```python
from build123d import *

# Parameters (mm, degrees)
SKETCH_1_R          = 1.65
EXTRUDE_1_DEPTH     = 4
CUT_EXTRUDE_1_DEPTH = 2
SKETCH_5_R          = 3.15
SKETCH_5_R_2        = 1.65
EXTRUDE_3_DEPTH     = 2.5
EXTRUDE_2_DEPTH     = 14.5
SKETCH_4_R          = 1.15
CUT_EXTRUDE_2_DEPTH = 13.5
CUT_EXTRUDE_3_DEPTH = 8.5
EXTRUDE_4_DEPTH     = 4
FILLET_1_R          = 3


with BuildPart() as part:
    # 草图1 → 凸台-拉伸1 (new body)
    with BuildSketch(Plane.XY):
        with BuildLine():
            Line((-24.466432563, 19.444503372), (0, 5))
            Line((0, 5), (24.466432563, 19.444503372))
            ThreePointArc((24.466432563, 19.444503372), (29.880062562, 18.138966358), (28.742325032, 12.687602311))
            Line((28.742325032, 12.687602311), (10, 0))
            Line((10, 0), (28.742325032, -12.687602311))
            ThreePointArc((28.742325032, -12.687602311), (29.880062562, -18.138966358), (24.466432563, -19.444503372))
            Line((24.466432563, -19.444503372), (0, -5))
            Line((0, -5), (-24.466432563, -19.444503372))
            ThreePointArc((-24.466432563, -19.444503372), (-29.880062562, -18.138966358), (-28.742325032, -12.687602311))
            Line((-28.742325032, -12.687602311), (-10, 0))
            Line((-10, 0), (-28.742325032, 12.687602311))
            ThreePointArc((-28.742325032, 12.687602311), (-29.880062562, 18.138966358), (-24.466432563, 19.444503372))
        make_face()
        with Locations((-26.5, 16)):
            Circle(SKETCH_1_R, mode=Mode.SUBTRACT)
        with Locations((26.5, 16)):
            Circle(SKETCH_1_R, mode=Mode.SUBTRACT)
        with Locations((26.5, -16)):
            Circle(SKETCH_1_R, mode=Mode.SUBTRACT)
        with Locations((-26.5, -16)):
            Circle(SKETCH_1_R, mode=Mode.SUBTRACT)
    extrude(amount=EXTRUDE_1_DEPTH)

    # 草图2 → 切除-拉伸1 (cut)
    with BuildSketch(Plane.XY.offset(4)):
        Polygon((-24.854551733, 18.85), (-28.145448267, 18.85), (-29.790896534, 16), (-28.145448267, 13.15), (-24.854551733, 13.15), (-23.209103466, 16), align=None)
        Polygon((28.145448267, 18.85), (24.854551733, 18.85), (23.209103466, 16), (24.854551733, 13.15), (28.145448267, 13.15), (29.790896534, 16), align=None)
        Polygon((28.145448267, -13.15), (24.854551733, -13.15), (23.209103466, -16), (24.854551733, -18.85), (28.145448267, -18.85), (29.790896534, -16), align=None)
        Polygon((-24.854551733, -13.15), (-28.145448267, -13.15), (-29.790896534, -16), (-28.145448267, -18.85), (-24.854551733, -18.85), (-23.209103466, -16), align=None)
    extrude(amount=-CUT_EXTRUDE_1_DEPTH, mode=Mode.SUBTRACT)

    # 草图5 → 凸台-拉伸3 (add)
    with BuildSketch(Plane(origin=(0, 0, 0), x_dir=(-1, 0, 0), z_dir=(0, 0, -1))):
        with Locations((26.5, 16)):
            Circle(SKETCH_5_R)
        with Locations((26.5, 16)):
            Circle(SKETCH_5_R_2, mode=Mode.SUBTRACT)
        with Locations((26.5, -16)):
            Circle(SKETCH_5_R)
        with Locations((26.5, -16)):
            Circle(SKETCH_5_R_2, mode=Mode.SUBTRACT)
        with Locations((-26.5, -16)):
            Circle(SKETCH_5_R)
        with Locations((-26.5, -16)):
            Circle(SKETCH_5_R_2, mode=Mode.SUBTRACT)
        with Locations((-26.5, 16)):
            Circle(SKETCH_5_R)
        with Locations((-26.5, 16)):
            Circle(SKETCH_5_R_2, mode=Mode.SUBTRACT)
    extrude(amount=EXTRUDE_3_DEPTH)

    # 草图3 → 凸台-拉伸2 (add, symmetric)
    with BuildSketch(Plane(origin=(0, 0, 0), x_dir=(0, 0, -1), z_dir=(1, 0, 0))):
        Polygon((0, -8.75), (0, -3.25), (-6.75, -3.25), (-8, -2), (-10, -2), (-10, -10), (-8, -10), (-6.75, -8.75), align=None)
    extrude(amount=EXTRUDE_2_DEPTH, both=True)

    # 草图4 → 切除-拉伸2 (cut, through all)
    with BuildSketch(Plane.XY.offset(10)):
        with Locations((-11.25, -6)):
            Circle(SKETCH_4_R)
        with Locations((11.25, -6)):
            Circle(SKETCH_4_R)
    extrude(amount=-CUT_EXTRUDE_2_DEPTH, mode=Mode.SUBTRACT)

    # 草图6 → 切除-拉伸3 (cut)
    with BuildSketch(Plane(origin=(0, 0, 0), x_dir=(-1, 0, 0), z_dir=(0, 0, -1))):
        Polygon((-10.066431948, -3.95), (-12.433568052, -3.95), (-13.617136104, -6), (-12.433568052, -8.05), (-10.066431948, -8.05), (-8.882863896, -6), align=None)
        Polygon((12.433568052, -3.95), (10.066431948, -3.95), (8.882863896, -6), (10.066431948, -8.05), (12.433568052, -8.05), (13.617136104, -6), align=None)
    extrude(amount=-CUT_EXTRUDE_3_DEPTH, mode=Mode.SUBTRACT)

    # 草图7 → 凸台-拉伸4 (add)
    with BuildSketch(Plane(origin=(0, 0, 0), x_dir=(-1, 0, 0), z_dir=(0, 0, -1))):
        with BuildLine():
            Line((17.5, -5.07711915), (40.5, -5.07711915))
            Line((40.5, -5.07711915), (40.5, -56))
            Line((40.5, -56), (17.5, -56))
            Line((17.5, -56), (17.5, -15.331657807))
            Line((17.5, -15.331657807), (24.466432563, -19.444503372))
            ThreePointArc((24.466432563, -19.444503372), (29.880062562, -18.138966358), (28.742325032, -12.687602311))
            Line((28.742325032, -12.687602311), (17.5, -5.07711915))
        make_face()
    extrude(amount=-EXTRUDE_4_DEPTH)

    # 圆角1
    fillet_1_edges = [part.edges().sort_by_distance(p)[0] for p in [
        (-40.5, -5.07711915, 2),
        (-40.5, -56, 2),
        (-17.5, -56, 2),
        (-17.5, -15.331657807, 2),
    ]]
    fillet(fillet_1_edges, radius=FILLET_1_R)


solid = part.part
```
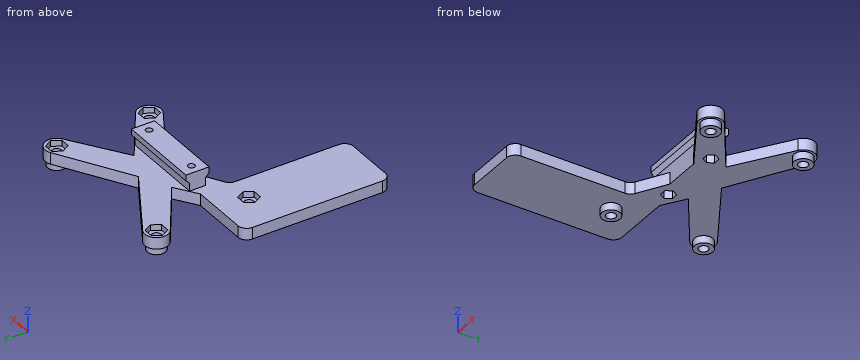
Check sheet for the modelled part. Datum: model origin and axes. Units: mm. Give positions to 0.01 mm unless a question says otherwise; leave off trailing zeros. Write each loop counter-clockwise with the first axis right and the second up, starting at its lowest first coordinate (ties: lowest second). Pieces come first, ordered by that corner, then holes.
Item 1: Cross-section at C-C (z = 5.25). Enter the section's corners in (x, y).
Item 2: Scan lines: L1, parallel to Y at x = 26.5, z = -1.05; L2, parallel to X at y = -16, z = 1.6; L3, parallel to Y at x = -26.5, z = 1.1. Record each from-to range of solid material in increasing order.
Item 3: Cross-section at D-D (x = -22). Enter the section's corners in (y, z), and give its area (3 significant figures).
Item 4: Gauge pin test, flat ends, axial feed: pin 1 (1.6 mm diameter, centred on x = -3.5, z = 9.5, fed in from +Y); pin 2 (3 mm diameter, centred on x = 27, y = -16.5, fed in from +Z); pin 3 (1 mm diameter, centred on x = 2, z = 9, fed in from -Y); pin 4 (2 mm diameter, centred on x = -26.5, y = 16, fed in from -Z) (3 decimals). Record the tip position at first contact, or that the pin passes through.
Item 5: Cross-section at A-A (z = -1.5). Enter the section's corners in (x, y).
Item 6: Cross-section at B-B (x = -11.25). Enter the section's corners in (y, z), and give its area (3 significant figures).
Report:
1. outline: (-14.5, -8.75) - (14.5, -8.75) - (14.5, -3.25) - (-14.5, -3.25) - close; hole (-13.62, -6) - (-12.43, -8.05) - (-10.07, -8.05) - (-8.88, -6) - (-10.07, -3.95) - (-12.43, -3.95) - close; hole (8.88, -6) - (10.07, -8.05) - (12.43, -8.05) - (13.62, -6) - (12.43, -3.95) - (10.07, -3.95) - close
2. L1: y = -19.15 to -17.65, -14.35 to -12.85, 12.85 to 14.35, 17.65 to 19.15
2. L2: x = -40.5 to -28.15, -24.85 to -17.31, 18.63 to 24.85, 28.15 to 30.5
2. L3: y = -56 to -17.65, -14.35 to -5.08, 11.17 to 14.35, 17.65 to 20
3. outline: (-56, 0) - (-5.08, 0) - (-5.08, 4) - (-56, 4) - close; (8.12, 0) - (17.99, 0) - (17.99, 4) - (8.12, 4) - close
3. area: 243 mm2
4. pin 1: stops at y = -2
4. pin 2: stops at z = 2
4. pin 3: stops at y = -10
4. pin 4: passes through
5. outline: circle Ø6.3 at (-26.5, -16); circle Ø6.3 at (-26.5, 16); circle Ø6.3 at (26.5, -16); circle Ø6.3 at (26.5, 16); hole circle Ø3.3 at (-26.5, -16); hole circle Ø3.3 at (-26.5, 16); hole circle Ø3.3 at (26.5, -16); hole circle Ø3.3 at (26.5, 16)
6. outline: (-11.64, 0) - (-8.05, 0) - (-8.05, 8.5) - (-7.15, 8.5) - (-7.15, 10) - (-10, 10) - (-10, 8) - (-8.75, 6.75) - (-8.75, 4) - (-11.64, 4) - close; (-4.85, 8.5) - (-3.95, 8.5) - (-3.95, 0) - (-0.85, 0) - (-0.85, 4) - (-3.25, 4) - (-3.25, 6.75) - (-2, 8) - (-2, 10) - (-4.85, 10) - close; (0.85, 0) - (11.64, 0) - (11.64, 4) - (0.85, 4) - close
6. area: 87.6 mm2
